Geometry: final body of the model. Coordinates: model frame, mm. Face numbers are marked on the shaded views. Round coordinates to 2 decimals unless told otherwise and drop trailing zeros. Write each loop counter-clockwise with the first axis right and the second up, starting at its lowest first coordinate (ties: lowest second). Pieces come first, ordered by that corner, then holes. Notation, with made-up numbers: M 55,-13.75 L 104,-13.75 A33 cw 104,21.25 Z; hole C 63.25,-6 d9. An arc over 180 degrees is marked long. Use one line per item in the form item = value. Start each with the question number.
Item 1: Section query B-B (z = 9.25). Return loops of the section in (x, y).
Item 2: Ray query, probe 1 along X at (y, z) = (1.75, 1); probe 2 along Y at (x, z) = (-10, 5.5); probe 3 along X at (y, z) = (-0.5, 3.75). Return the intervals inside material, ascending.
Item 3: Section query C-C (y = 0). Return loops of the section in (x, z), and give its area (3 significant figures).
Item 4: Section query A-A (x = 0). Return loops of the section in (y, z), and give its area (3 significant figures).
Item 5: Pull-direction query (Y, two-part tool) for the marked faces 1, 2 and 3; classes: pulls with the +Y half, pulls with the -Y half, needs draft (parallel to the pull), parting line crosses it, or undercut.
Item 6: Section query D-D (x = 9). Return loops of the section in (y, z).
from build123d import *

# Parameters (mm, degrees)
SKETCH_1_R      = 2
EXTRUDE_1_DEPTH = 10


with BuildPart() as part:
    # 草图1 → 凸台-拉伸1 (new body)
    with BuildSketch(Plane.XY):
        with BuildLine():
            Line((-10, 4), (10, 4))
            ThreePointArc((10, 4), (14, 0), (10, -4))
            Line((10, -4), (-10, -4))
            ThreePointArc((-10, -4), (-14, 0), (-10, 4))
        make_face()
        with Locations((-10, 0)):
            Circle(SKETCH_1_R, mode=Mode.SUBTRACT)
        with Locations(Location((10, 0, 0), (0, 0, 180))):
            Circle(SKETCH_1_R, mode=Mode.SUBTRACT)
        Circle(SKETCH_1_R, mode=Mode.SUBTRACT)
    extrude(amount=EXTRUDE_1_DEPTH)


solid = part.part
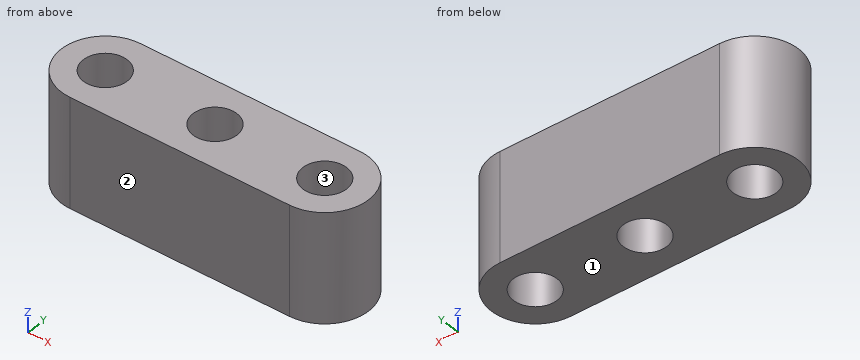
Working result:
q1.outline = M -10,-4 L 10,-4 A4 ccw 10,4 L -10,4 A4 ccw Z; hole C -10,0 d4; hole C 0,0 d4; hole C 10,0 d4
q2.probe_1 = -13.6 to -10.97, -9.03 to -0.97, 0.97 to 9.03, 10.97 to 13.6
q2.probe_2 = -4 to -2, 2 to 4
q2.probe_3 = -13.97 to -11.94, -8.06 to -1.94, 1.94 to 8.06, 11.94 to 13.97
q3.outline = M -14,0 L -12,0 L -12,10 L -14,10 Z; M -8,0 L -2,0 L -2,10 L -8,10 Z; M 2,0 L 8,0 L 8,10 L 2,10 Z; M 12,0 L 14,0 L 14,10 L 12,10 Z
q3.area = 160 mm²
q4.outline = M -4,0 L -2,0 L -2,10 L -4,10 Z; M 2,0 L 4,0 L 4,10 L 2,10 Z
q4.area = 40.0 mm²
q5.face_1 = needs draft
q5.face_2 = pulls with the -Y half
q5.face_3 = undercut
q6.outline = M -4,0 L -1.73,0 L -1.73,10 L -4,10 Z; M 1.73,0 L 4,0 L 4,10 L 1.73,10 Z
